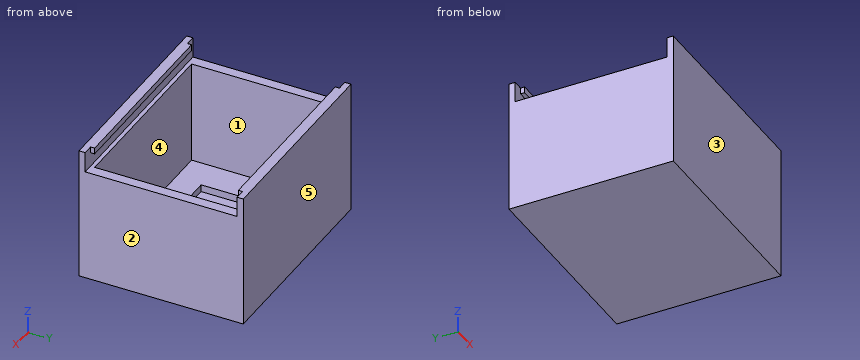
from build123d import *

# Parameters (mm, degrees)
SKETCH_W        = 90
SKETCH_H        = 70
PAD_DEPTH       = 60
THICKNESS_T     = 5
SKETCH001_W     = 45
SKETCH001_H     = 45
POCKET_DEPTH    = 3.5
POCKET001_DEPTH = 3.5
SKETCH002_W     = 74
SKETCH002_H     = 10
POCKET002_DEPTH = 5
SKETCH003_W     = 74
SKETCH003_H     = 10
POCKET003_DEPTH = 5
SKETCH004_W     = 74
SKETCH004_H     = 7
POCKET004_DEPTH = 90


with BuildPart() as part:
    # Sketch → Pad (new body)
    with BuildSketch(Plane.XY):
        Rectangle(SKETCH_W, SKETCH_H)
    extrude(amount=PAD_DEPTH)

    # Thickness
    thickness_openings = [part.faces().sort_by_distance(p)[0] for p in [
        (0, 0, 60),
    ]]
    offset(amount=THICKNESS_T, openings=thickness_openings, kind=Kind.INTERSECTION)

    # Sketch001 (on Face5 of Thickness) → Pocket (cut)
    with BuildSketch(Plane.XY):
        with Locations((-7.5, 0)):
            Rectangle(SKETCH001_W, SKETCH001_H)
    extrude(amount=-POCKET_DEPTH, mode=Mode.SUBTRACT)

    # Sketch001 (on Face5 of Thickness) → Pocket001 (cut)
    with BuildSketch(Plane.XY):
        with Locations((-7.5, 0)):
            Rectangle(SKETCH001_W, SKETCH001_H)
    extrude(amount=-POCKET001_DEPTH, mode=Mode.SUBTRACT)

    # Sketch002 (on Face12 of Pocket001) → Pocket002 (cut)
    with BuildSketch(Plane(origin=(-50, 0, 0), x_dir=(0, -1, 0), z_dir=(-1, 0, 0))):
        with Locations((0, 55)):
            Rectangle(SKETCH002_W, SKETCH002_H)
    extrude(amount=-POCKET002_DEPTH, mode=Mode.SUBTRACT)

    # Sketch003 (on Face18 of Pocket002) → Pocket003 (cut)
    with BuildSketch(Plane.YZ.offset(50)):
        with Locations((0, 55)):
            Rectangle(SKETCH003_W, SKETCH003_H)
    extrude(amount=-POCKET003_DEPTH, mode=Mode.SUBTRACT)

    # Sketch004 (on Face3 of Pocket003) → Pocket004 (cut)
    with BuildSketch(Plane(origin=(-45, 0, 0), x_dir=(0, -1, 0), z_dir=(-1, 0, 0))):
        with Locations((0, 53.5)):
            Rectangle(SKETCH004_W, SKETCH004_H)
    extrude(amount=-POCKET004_DEPTH, mode=Mode.SUBTRACT)


solid = part.part
Could you check a few things on this model? Use its own coordinates, in mm. Face numbers are marked on the shaded views. A direction names the side the tool comes from. Give positions to 0.01 mm unless a question says otherwise; leave off trailing zeros. Write each loop counter-clockwise with the first axis right and the second up, starting at its lowest first coordinate (ties: lowest second). Pieces come first, ordered by that corner, then holes. Notation, with made-up numbers: (59, 69.25) - (77, 69.25) arc R9 ccw to (77, 78.25) - close; hole circle Ø11 at (-1, 43). An arc over 180 degrees is marked (long way). Use CSV: the item, a comma, the result in double quotes. Start each with the question number.
Item 1: I want a section at A-A, the plane z = 7.5. Please give me the cut outline in (x, y), then the cut area to 3 significant figures.
Item 2: I want a section at D-D, the plane x = 13. Please give me the cut outline in (y, z).
Item 3: If I drill on line 1 along Y through (x, z) = (-25.5, 25); line 2 along Z through (x, y) = (-9, 36); line 3 along X through (y, z) = (-16, 26.5), over which ranges is the centre line in solid material (lowest first)?
Item 4: For the marked faces 4 and 5, which set-ups out of +Z, -Z, +X, -X, +Y, -Y let a thin tool reach every point of the face, with its end or its side?
Item 5: If we mould it in two halves opening along Y, with no side actions, what happens to the marked faces 1, 2 and 3? For each: pulls with the +Y half, pulls with the -Y half, needs draft (parallel to the pull), parting line crosses it, or undercut.
Item 6: I want a section at C-C, the plane y = -11. Please give me the cut outline in (x, z), then the cut area to 4 significant figures.
Item 7: I want a section at B-B, the plane x = 34.5. Please give me the cut outline in (y, z).
Item 8: I'm going to push flat-ended pins straight in: pin 1 (22.5 mm diameter, centred on x = -7, y = 1, fed in from +Z); pin 2 (0.6 mm diameter, centred on y = 36, z = 58.5, fed in from +X); pin 3 (21 mm diameter, centred on x = 17, y = -7, fed in from +Z). Where does each tip first touch, or does it pass through?
Findings:
1,outline,"(-50, -40) - (50, -40) - (50, 40) - (-50, 40) - close; hole (-45, -35) - (45, -35) - (45, 35) - (-45, 35) - close"
1,area,"1,700 mm2"
2,outline,"(-40, -5) - (40, -5) - (40, 60) - (35, 60) - (35, 57) - (37, 57) - (37, 50) - (35, 50) - (35, 0) - (22.5, 0) - (22.5, -3.5) - (-22.5, -3.5) - (-22.5, 0) - (-35, 0) - (-35, 50) - (-37, 50) - (-37, 57) - (-35, 57) - (-35, 60) - (-40, 60) - close"
3,line 1,"y = -40 to -35, 35 to 40"
3,line 2,"z = -5 to 50, 57 to 60"
3,line 3,"x = -50 to -45, 45 to 50"
4,face 4,"+Z"
4,face 5,"+Z, -Z, +X, -X, +Y"
5,face 1,"undercut"
5,face 2,"needs draft"
5,face 3,"pulls with the -Y half"
6,outline,"(-50, -5) - (50, -5) - (50, 50) - (45, 50) - (45, 0) - (15, 0) - (15, -3.5) - (-30, -3.5) - (-30, 0) - (-45, 0) - (-45, 50) - (-50, 50) - close"
6,area,"842.5 mm2"
7,outline,"(-40, -5) - (40, -5) - (40, 60) - (35, 60) - (35, 57) - (37, 57) - (37, 50) - (35, 50) - (35, 0) - (-35, 0) - (-35, 50) - (-37, 50) - (-37, 57) - (-35, 57) - (-35, 60) - (-40, 60) - close"
8,pin 1,"stops at z = -3.5"
8,pin 2,"stops at x = 45"
8,pin 3,"stops at z = 0"
